For this review, take the finished solid that the model builds, in its own axes (mm). A direction names the side the tool comes from. Coordinates: 2 decimals unless noted, no trailing zeros. Write each loop counter-clockwise with the first axis right and the second up, starting at its lowest first coordinate (ties: lowest second). Pieces come first, ordered by that corner, then holes. Notation, with made-up numbers: (40.5, 84) -> (44.5, 84) arc R23 ccw to (44.5, 98) -> close; hole circle Ø10 at (58, 58.5). An arc over 180 degrees is marked (long way). One line per item, written item: value. Start each with the question number.
1) Add section A-A (z = 0). State the section outline as (x, y) points (3 decimals).
2) Add section C-C (y = -16). State the section outline as (x, z) points (3 decimals).
3) Add section D-D (y = -22.5). State the section outline as (x, z) points.
4) Mouldability with a two-part tool opening along Z and no side actions: class faces 4 (the cylindrical face through (-1.93, -0.28, -2.52)), 5 (the flat face through (1, 20.32, -1)), 6 (the flat face through (0, 25, -0.75)) as released by +Z, released by -Z, zero draft, split by the parting line, or undercut.
5) For pin 1 Ø0.7 at (x, y) = (0, -25.5) entering from -Z; pin 2 Ø3 at (x, z) = (-2.5, -2) entering from +Y; pin 3 Ø2 at (x, y) = (2.5, -9) entering from +Z, all flat-tipped, find the tip position at first contact; note any pin that passes through.
6) Add section B-B (x = 0). State the section outline as (y, z) points (3 decimals).
7) Machinability: for faces 1 (the flat face through (0, -25, 0.75)), 2 (the flat face through (0, 25, 0.75)), 3 (the flat face through (1, -20.32, -1)), which of the approach directions +Z, -Z, +X, -X, +Y, -Y give a long, thin tool a straight path to every point of the face, cutting with its end or side? Answer none if there is none.
8) For probe 1 along Y at (x, z) = (-2, 1.25); probe 2 along X at (y, z) = (-7, -0.25); probe 3 along Z at (x, y) = (0.5, 6), list the stretches that pass through material, from the lowest coordinate up. Write a range as from..to.
from build123d import *

# Parameters (mm, degrees)
BOSS_EXTRUDE1_DEPTH      = 20.32
BOSS_EXTRUDE1_DEPTH_BACK = 20.32
SKETCH1_R                = 3.175
SKETCH2_R                = 1
BOSS_EXTRUDE2_DEPTH      = 6.35
CUT_EXTRUDE1_DEPTH       = 6.35


with BuildPart() as part:
    # Sketch1 → Boss-Extrude1 (new, two sides: drawn at the far end of the back side and taken through both)
    with BuildSketch(Plane(origin=(0, 0, 0), x_dir=(1, 0, 0), z_dir=(0, 1, 0)).offset(-BOSS_EXTRUDE1_DEPTH_BACK)):
        with Locations(Location((0, 0, 0), (0, 0, 270))):
            Circle(SKETCH1_R)
    extrude(amount=BOSS_EXTRUDE1_DEPTH + BOSS_EXTRUDE1_DEPTH_BACK)

    # Sketch2 → Boss-Extrude2 (add)
    with BuildSketch(Plane(origin=(0, 20.32, 0), x_dir=(1, 0, 0), z_dir=(0, 1, 0))):
        with Locations(Location((0, 0, 0), (0, 0, 270))):
            Circle(SKETCH2_R)
    boss_extrude2 = extrude(amount=BOSS_EXTRUDE2_DEPTH)

    # Sketch3 → Cut-Extrude1 (cut)
    with BuildSketch(Plane(origin=(0, 23.320000096, 0), x_dir=(1, 0, 0), z_dir=(0, 1, 0))):
        with BuildLine():
            ThreePointArc((0.661437828, 0.75), (0, 1), (-0.661437828, 0.75))
            Line((-0.661437828, 0.75), (0.661437828, 0.75))
        make_face()
        with BuildLine():
            Line((0.661437828, -0.75), (-0.661437828, -0.75))
            ThreePointArc((-0.661437828, -0.75), (0, -1), (0.661437828, -0.75))
        make_face()
    cut_extrude1 = extrude(amount=CUT_EXTRUDE1_DEPTH, mode=Mode.SUBTRACT)

    # Mirror1: Boss-Extrude2, Cut-Extrude1 across plane
    add(boss_extrude2.mirror(Plane.ZX))
    add(cut_extrude1.mirror(Plane.ZX), mode=Mode.SUBTRACT)


solid = part.part
Numbers:
1. outline: (-3.175, -20.32) -> (-1, -20.32) -> (-1, -26.67) -> (1, -26.67) -> (1, -20.32) -> (3.175, -20.32) -> (3.175, 20.32) -> (1, 20.32) -> (1, 26.67) -> (-1, 26.67) -> (-1, 20.32) -> (-3.175, 20.32) -> close
2. outline: circle Ø6.35 at (0, 0)
3. outline: circle Ø2 at (0, 0)
4. face 4: split by the parting line
4. face 5: zero draft
4. face 6: released by -Z
5. pin 1: z = -0.75
5. pin 2: y = 20.32
5. pin 3: z = 2.8
6. outline: (-26.67, -0.75) -> (-23.32, -0.75) -> (-23.32, -1) -> (-20.32, -1) -> (-20.32, -3.175) -> (20.32, -3.175) -> (20.32, -1) -> (23.32, -1) -> (23.32, -0.75) -> (26.67, -0.75) -> (26.67, 0.75) -> (23.32, 0.75) -> (23.32, 1) -> (20.32, 1) -> (20.32, 3.175) -> (-20.32, 3.175) -> (-20.32, 1) -> (-23.32, 1) -> (-23.32, 0.75) -> (-26.67, 0.75) -> close
7. face 1: +Z, +X, -X, -Y
7. face 2: +Z, +X, -X, +Y
7. face 3: -Y
8. probe 1: -20.32..20.32
8. probe 2: -3.17..3.17
8. probe 3: -3.14..3.14
